Autodesk Inventor part; units mm, degrees
ref_plane "Work Plane3" through (-50, 0, 0) normal (-1, 0, 0) x (0, 0, 1)
ref_plane "YZ Plane" through (0, 0, 0) normal (1, 0, 0) x (0, 1, 0)
ref_plane "XZ Plane" through (0, 0, 0) normal (0, 1, 0) x (-1, 0, 0)
ref_plane "Work Plane3" through (-50, 0, 0) normal (-1, 0, 0) x (0, 0, 1)
sketch "Sketch6" plane through (-50, 0, 0) normal (-1, 0, 0) x (0, 0, 1)
  arc A0 (-92.5702, 77.4165) -> (-109.8479, 59.8803) centre (-96.1815, 63.695) ccw
  line L0 (-70.536, 69.486) -> (-92.5702, 77.4165)
  line L1 (44.1213, 28.2183) -> (-70.536, 69.486)
  arc A1 (53.2724, 20) -> (44.1213, 28.2183) centre (36.052, 10.0292) ccw
  arc A2 (53.2724, 20) -> (69.1541, 1.9881) centre (80.7478, 28.2183) ccw
  arc A3 (69, 0) -> (69.1541, 1.9881) centre (69, 1) ccw
  line L2 (45, 0) -> (69, 0)
  line L3 (45, 15) -> (45, 0)
  arc A4 (45, 15) -> (42, 18) centre (42, 15) ccw
  line L4 (3, 18) -> (42, 18)
  arc A5 (3, 18) -> (0, 15) centre (3, 15) ccw
  line L5 (0, 0) -> (0, 15)
  line L6 (0, 0) -> (-57.7, 0)
  line L7 (-57.7, 0) -> (-57.7, 12)
  arc A6 (-57.7, 12) -> (-60.7, 15) centre (-60.7, 12) ccw
  line L8 (-60.7, 15) -> (-101.1648, 15)
  arc A7 (-104.1648, 18.006) -> (-101.1648, 15) centre (-101.1648, 18) ccw
  arc A8 (-104.1648, 18.006) -> (-109.8479, 59.8803) centre (-258.9764, 18.3179) ccw
extrude "Extrusion2" add sketch "Sketch6" along normal blind 2
sketch "Sketch7" plane through (-50, 0, 0) normal (1, 0, 0) x (0, 0, -1)
  circle A0 centre (75.7329, 49.2486) radius 2.5
  circle A1 centre (-53.2724, 6.5547) radius 1.5
  point P0 (0, 0)
extrude "Extrusion3" cut sketch "Sketch7" against normal blind 10
chamfer "Chamfer1" distance 2 angle 45 1 edges at (-50, 49.2486, -73.2329)
chamfer "Chamfer2" distance 1 angle 45 1 edges at (-50, 6.5547, 54.7724)
properties part number "tampa frontal - corpo"
Geometry check sheet. Reference: the model listing, model coordinates, mm. A direction names the side the tool comes from. Coordinates: 2 decimals unless noted, no trailing zeros. Loops run counter-clockwise (first coordinate to the right, second up) from the corner with the lowest first, then second, coordinate; pieces in that order, holes last. Notation, with made-up numbers: (42.25, -10) - (59.25, -10) arc R5 cw to (59.25, -5) - close; hole circle Ø4 at (68, 46). An arc over 180 degrees is marked (long way). Use one line per item in the form item = value. Start each with the question number.
Item 1: Tool access check on faces 1 (the face through (-50.99, 17.1, 0.86)), 2 (the face through (-50.99, 14.14, -58.6)). Record the directions out of +Z, -Z, +X, -X, +Y, -Y that give a thin tool (end or side, any length) a straight path to the whole face; none if there is none.
Item 2: Gauge pin test, flat ends, axial feed: pin 1 (1 mm diameter, centred on x = -51.5, z = -71.5, fed in from -Y); pin 2 (1 mm diameter, centred on x = -50.5, z = 31.5, fed in from -Y). Record the tip position at first contact, or that the pin passes through.
Item 3: Mould release check, pull along Z, two halves, no side actions. Record for faces 3 (the face through (-52, 31, -41)), 4 (the face through (-51.49, 5.64, 54.46)), 5 (the face through (-50.99, 17.14, 44.1)), 6 (the face through (-50.99, 39.43, -105.61)): +Z half, -Z half, draft (parallel to the pull), parting line (faces both ways), or undercut.
Item 4: Section check B-B, the plane y = 39. Enter the section's corners in (x, z).
Item 5: Section check A-A, the plane x = -50.4. Enter the section's corners in (y, z).
Item 6: Section check C-C, the plane z = 19.5. Enter the section's corners in (x, y), and give its area (3 significant figures).
Item 7: Thickness scan on probe 1 along Z at (x, y) = (-51.45, 20); probe 2 along Y at (x, z) = (-51, -72); probe 3 along Y at (x, z) = (-51.7, -95.5). Record the ranges inside material, lowest first.
Computed:
q1.face_1 = +X, -X, -Y
q1.face_2 = -Z, +X, -X, -Y
q2.pin_1 = 15
q2.pin_2 = 18
q3.face_3 = draft
q3.face_4 = undercut
q3.face_5 = undercut
q3.face_6 = -Z half
q4.outline = (-52, -105.55) - (-50, -105.55) - (-50, 14.17) - (-52, 14.17) - close
q5.outline = (0, -57.7) - (12, -57.7) arc R3 cw to (15, -60.7) - (15, -101.16) arc R3 ccw to (18.01, -104.16) arc R154.81 cw to (59.88, -109.85) arc R14.19 ccw to (77.42, -92.57) - (69.49, -70.54) - (28.22, 44.12) arc R19.9 ccw to (20, 53.27) arc R28.68 cw to (1.99, 69.15) arc R1 ccw to (0, 69) - (0, 45) - (15, 45) arc R3 cw to (18, 42) - (18, 3) arc R3 cw to (15, 0) - (0, 0) - close; hole circle Ø4.2 at (6.55, 53.27); hole circle Ø8.2 at (49.25, -75.73)
q6.outline = (-52, 18) - (-50, 18) - (-50, 37.08) - (-52, 37.08) - close
q6.area = 38.2 mm2
q7.probe_1 = -104.17 to 53.27
q7.probe_2 = 15 to 70.01
q7.probe_3 = 15 to 77.87
